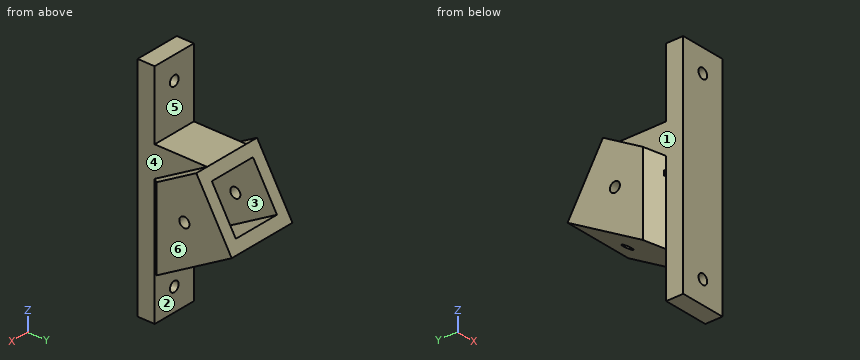
Autodesk Inventor part; units mm, degrees
ref_plane "YZ Plane" through (0, 0, 0) normal (1, 0, 0) x (0, 1, 0)
ref_plane "XZ Plane" through (0, 0, 0) normal (0, 1, 0) x (-1, 0, 0)
ref_plane "XY Plane" through (0, 0, 0) normal (0, 0, 1) x (1, 0, 0)
sketch "Sketch1" plane through (0, 0, 0) normal (1, 0, 0) x (0, 1, 0)
  line L0 (0, 0) -> (29.1856, 16.8503)
  line L1 (29.1856, 16.8503) -> (48.8706, -17.2451)
  line L2 (0, -71.1236) -> (0, 36.9987)
  line L3 (48.8706, -17.2451) -> (0, -45.4606)
  line L4 (0, 0) -> (0, -45.4606)
  line L5 (32.9956, 10.2512) -> (0, -8.7988) construction
  dimension "d0" = 39.37
  dimension "d1" = 60
  dimension "d5" = 7.62
  dimension "d6" = 38.1
extrude "Extrusion1" add sketch "Sketch1" along normal mid plane 39.37
sketch "Sketch2" plane through (-19.685, 29.1856, 16.8503) normal (0, 0.8660254, 0.5) x (1, 0, 0)
  line L0 (0, 0) -> (39.37, 0) construction
  line L1 (39.37, 0) -> (39.37, 39.37) construction
  line L2 (0, 0) -> (39.37, 39.37) construction
  line L3 (39.37, 39.37) -> (0, 39.37) construction
  line L4 (0, 39.37) -> (39.37, 0) construction
  line L5 (6.35, 6.35) -> (33.02, 6.35)
  line L6 (33.02, 6.35) -> (33.02, 33.02)
  line L7 (33.02, 33.02) -> (6.35, 33.02)
  line L8 (6.35, 33.02) -> (6.35, 6.35)
  line L9 (6.35, 6.35) -> (33.02, 33.02) construction
  line L10 (33.02, 6.35) -> (6.35, 33.02) construction
  point P0 (19.685, 0)
  point P1 (19.685, 19.685)
  dimension "d7" = 26.67
extrude "Extrusion2" cut sketch "Sketch2" against normal blind 38.1
sketch "Sketch3" plane through (0, 0, 0) normal (1, 0, 0) x (0, 1, 0)
  line L0 (29.1856, 16.8503) -> (0, 0)
  line L1 (0, 0) -> (0, -45.4606)
  line L2 (0, -45.4606) -> (48.8706, -17.2451)
  line L3 (12.7, -30.7959) -> (0, -8.7988)
  line L4 (32.3606, 11.351) -> (0, -7.3323)
  line L5 (0, 0) -> (0, -45.4606)
  line L6 (29.1856, 16.8503) -> (15.6348, 16.8503) construction
  line L7 (0, 0) -> (29.1856, 16.8503)
  line L8 (0, 0) -> (0, 54.9503)
  line L9 (48.8706, -17.2451) -> (0, -45.4606)
  line L10 (0, -45.4606) -> (0, -70.8606)
  line L11 (0, -109.2236) -> (0, 87.7987)
  line L12 (0, 54.9503) -> (-9.525, 54.9503)
  line L13 (-9.525, 54.9503) -> (-9.525, -70.8606)
  line L14 (-9.525, -70.8606) -> (0, -70.8606)
  point P0 (1.0999, -13.335)
  point P1 (0, -15.24)
  point P2 (0, -8.7988)
  dimension "d10" = 38.1
  dimension "d11" = 25.4
  dimension "d12" = 9.525
  dimension "supportBaseLength" = 125.8109
extrude "Extrusion3" add sketch "Sketch3" along normal mid plane 25.4
sketch "Sketch5" plane through (0, 0, 0) normal (1, 0, 0) x (0, 1, 0)
  line L0 (0, 0) -> (29.1856, 16.8503)
  line L1 (0, 54.9503) -> (0, 0)
  line L2 (29.1856, 16.8503) -> (48.8706, -17.2451)
  line L3 (29.1856, 16.8503) -> (0, 16.8503)
  line L4 (0, 0) -> (29.1856, 16.8503)
extrude "Extrusion5" add sketch "Sketch5" along normal mid plane 25.4
sketch "Sketch4" plane through (0, 0, 0) normal (0, 0, 1) x (1, 0, 0)
  line L0 (19.685, 48.8706) -> (-19.685, 48.8706)
  line L1 (19.685, 0) -> (19.685, 48.8706)
  line L2 (19.685, 0) -> (12.7, 0)
  line L3 (12.7, 0) -> (-12.7, 0)
  line L4 (-12.7, 0) -> (-19.685, 0)
  line L5 (-19.685, 48.8706) -> (-19.685, 0)
  line L6 (-12.7, 0) -> (-12.7, -9.525)
  line L7 (12.7, -9.525) -> (-12.7, -9.525)
  line L8 (12.7, -9.525) -> (12.7, 0)
  line L9 (-12.7, 0) -> (-19.685, 6.985)
  line L10 (-19.685, 48.8706) -> (-19.685, 0)
  line L11 (-19.685, 6.985) -> (-19.685, 0)
  line L12 (0, 0) -> (0, 48.8706) construction
  line L13 (12.7, 0) -> (19.685, 0)
  line L14 (12.7, 0) -> (19.685, 6.985)
  line L15 (19.685, 6.985) -> (19.685, 0)
  dimension "d15" = 45
extrude "Extrusion4" cut sketch "Sketch4" against normal up to surface (125.8109 mm away) from surface at 54.9503 contours L1 L2 L14 | L9 L4 L5
sketch "Sketch6" plane through (-12.7, 0, 54.9503) normal (0, 1, 0) x (1, 0, 0)
  line L0 (25.4, 125.8109) -> (0, 125.8109) construction
  line L1 (12.7, 125.8109) -> (12.7, 0) construction
  line L2 (25.4, 0) -> (0, 0) construction
  point P0 (12.7, 54.9503)
  point P1 (12.7, 113.1109)
  point P2 (12.7, 12.7)
  dimension "d21" = 12.7
  dimension "d22" = 12.7
hole "Hole1" at (0, 0, -58.1606) at (0, 0, 42.2503) direction (0, -1, 0) diameter 5.6134 end through all
sketch "Sketch9" plane through (0, 0, 0) normal (1, 0, 0) x (0, 1, 0)
  line L0 (0.635, -6.9657) -> (0.635, -9.8987)
  line L1 (0.635, -9.8987) -> (12.7, -30.7959)
  line L2 (45.6956, -11.7459) -> (12.7, -30.7959)
  line L3 (32.3606, 11.351) -> (45.6956, -11.7459)
  line L4 (32.3606, 11.351) -> (0.635, -6.9657)
  line L5 (39.0281, -0.1974) -> (6.0325, -19.2474) construction
  line L6 (0.635, -9.8987) -> (12.7, -30.7959) construction
  circle A0 centre (22.5303, -9.7224) radius 2.8067
  point P0 (0, 0)
  dimension "d30" = 5.6134
extrude "Extrusion6" cut sketch "Sketch9" along normal through all both and the other way through all contours A0
sketch "Sketch10" plane through (-19.685, 48.8706, -17.2451) normal (0, 0.5, -0.8660254) x (1, 0, 0)
  line L0 (6.35, 0) -> (33.02, 0) construction
  line L1 (19.685, 0) -> (19.685, 77.7875) construction
  point P0 (19.685, 33.7006)
  point P1 (19.685, 19.05)
  dimension "d33" = 19.05
hole "Hole2" at (0, 32.3728, -26.7701) direction (0, -0.5, 0.8660254) diameter 5.6134 depth 6.35
equation "\"d0\" = widthToSupportExtrusion"
equation "\"d1\" = attachementAngle"
equation "\"d6\" = insertDepth"
equation "\"d2\" = widthToSupportExtrusion"
equation "\"d7\" = insertForExtrusion"
equation "\"d8\" = insertDepth"
equation "\"d10\" = lenghtUnderBrace"
equation "\"d11\" = backLength"
equation "\"d12\" = supportBaseDepth"
equation "\"d13\" = supportBaseWidth"
equation "\"d19\" = supportBaseWidth"
equation "\"attachementAngle\" = 60deg"
equation "\"extrusionSize\" = 25.4"
equation "\"wallThickness\" = 6.35"
equation "\"slipClearance\" = 0.635"
equation "\"insertForExtrusion\" = extrusionSize + 2 * slipClearance"
equation "\"widthToSupportExtrusion\" = insertForExtrusion + 2 * wallThickness"
equation "\"insertDepth\" = 38.1"
equation "\"supportBaseWidth\" = 25.4"
equation "\"supportBaseDepth\" = 9.525"
equation "\"supportHoleDistanceFromEnd\" = 12.7"
equation "\"lenghtUnderBrace\" = 38.1"
equation "\"backLength\" = 25.4"
properties part number "60DegreeAttachementV03"
Work out the finished part from the listing and answer in its coordinate system (mm). Face numbers are marked on the shaded views. A direction names the side the tool comes from. Give positions to 0.01 mm unless a question says otherwise; leave off trailing zeros. Order: outer loops, then holes, each group sorted by start corner. A loop starts at its lowest first (then second) coordinate and runs counter-clockwise, first axis right, second up. Notation, with made-up numbers: M -6,41 L 3,41 A27 cw 3,68 Z; hole C 38.5,-24.5 d2. An arc over 180 degrees is marked long. Return JSON: item names as keys, results as strings.
Q1. The mould has two halves that part along X. Classify the marked faces 1, 2 and 3: pulls with the +X half, pulls with the -X half, needs draft (parallel to the pull), parting line crosses it, or undercut.
Answer below:
{"face 1": "pulls with the -X half", "face 2": "needs draft", "face 3": "undercut"}
Q2. Find section A-A, the plane x = 0. Write down the section's boundary in (y, z) (3 decimals), and give its area (3 significant figures).
Answer below:
{"outline": "M -9.525,-70.861 L 0,-70.861 L 0,-60.967 L -9.525,-60.967 Z; M -9.525,-55.354 L 0,-55.354 L 0,-45.461 L 29.942,-28.173 L 26.767,-22.674 L 12.698,-30.797 L 0,-8.803 L 0,-7.332 L 32.361,11.351 L 29.186,16.85 L 0,16.85 L 0,39.444 L -9.525,39.444 Z; M -9.525,45.057 L 0,45.057 L 0,54.95 L -9.525,54.95 Z; M 31.628,-19.867 L 34.803,-25.367 L 48.871,-17.245 L 45.696,-11.746 Z", "area": "2,060 mm^2"}
Q3. Find section C-C, the plane z = 43. Write down the section's boundary in (x, y) (3 decimals), and give its area (3 significant figures).
Answer below:
{"outline": "M -12.7,-9.525 L -2.705,-9.525 L -2.705,0 L -12.7,0 Z; M 2.705,-9.525 L 12.7,-9.525 L 12.7,0 L 2.705,0 Z", "area": "190 mm^2"}
Q4. Which of the six approach directions +Z, -Z, +X, -X, +Y, -Y give full straight-line access (tool end or side, diameter ignored) to the marked faces 4, 5 and 6?
Answer below:
{"face 4": "+Z, +X, -Y", "face 5": "+Z, +X, -X, +Y", "face 6": "+Z, -Z, +X, +Y, -Y"}
Q5. Find the intervals of material crossed by line 1 along Z through (x, y) = (-2, -5); line 2 along X through (y, z) = (18, -22) (3 decimals); line 3 along Y through (x, z) = (3, -54.5) (3 decimals), in increasing order. Write a range as [from, to].
Answer below:
{"line 1": "z = [-70.86, -60.13], [-56.19, 40.28], [44.22, 54.95]", "line 2": "x = [-19.685, -13.335], [13.335, 19.685]", "line 3": "y = [-9.525, 0]"}
Q6. Find section B-B, the plane y = 10. Write down the section's boundary in (x, z) (1 decimal).
Answer below:
{"outline": "M -19.7,-39.7 L 19.7,-39.7 L 19.7,5.8 L 12.7,5.8 L 12.7,16.9 L -12.7,16.9 L -12.7,5.8 L -19.7,5.8 Z; hole M -13.3,-26.1 L 13.3,-26.1 L 13.3,-1.6 L -13.3,-1.6 Z"}
Q7. Each of these flat-tipped pins is pushed along its axis until it touches: pin 1 (1 mm diameter, centred on x = 10, y = 24.5, fed in from -Z); pin 2 (1.5 mm diameter, centred on y = -1, z = 17.5, fed in from +X); pin 3 (4 mm diameter, centred on x = -10, y = 11.5, fed in from -Z); pin 4 (9 mm diameter, centred on y = 22.53, z = -9.72, fed in from -X) (3 decimals). Where does it stop, or does it pass through?
Answer below:
{"pin 1": "stops at z = -31.6", "pin 2": "stops at x = 12.7", "pin 3": "stops at z = -39.98", "pin 4": "stops at x = -19.685"}
Q8. Find section D-D, the plane x = 17. Write down the section's boundary in (y, z).
Answer below:
{"outline": "M 4.3,-42.98 L 48.87,-17.25 L 29.19,16.85 L 4.3,2.48 Z; hole C 22.53,-9.72 d5.61"}
